Design review of the part shown in the three views and the two pictorial views. Dimensions are in mm from the part's minimum x, y and z. A direction names the side the tool comes from. Round coordinates to 2 decimals unless told otherwise and drop trailing zeros. Order: outer loops, then holes, each group sorted by start corner. A loop starts at its lowest first (then second) coordinate and runs counter-clockwise, first axis right, second up. Notation, with made-up numbers: (0.25, 79.5) - (40.25, 79.5) arc R27 cw to (40.25, 114.5) - close; hole circle Ø3 at (61.25, 9). An arc over 180 degrees is marked (long way). One line per question, with ' | ' between items. Start each with the question number.
Item 1: Add section A-A on z = 20.75. State the section outline as (x, y) points.
Item 2: Add section B-B on y = 96.5. State the section outline as (x, z) points, and give its area (3 significant figures).
Item 3: Add section C-C on x = 111. State the section outline as (y, z) points.
Item 4: Tool access review of the marked faces 1 and 2: name each direction out of +Z, -Z, +X, -X, +Y, -Y from which nothing blocks a thin tool from reaching the whole face with its end or side.
Item 5: Insertion check: pin 1 Ø4 at (x, y) = (143.5, 77.5) entering from +Z; pin 2 Ø8 at (x, z) = (82.5, 9) entering from +Y; pin 3 Ø2 at (x, z) = (116, 1.5) entering from +Y. Each pin has a flat end and moves straight along its axis. Give the tip position at first contact, or say it passes through.
Item 6: For L1, parallel to X at y = 14.5, z = 2.25; L2, parallel to X at y = 124, z = 12.5; L3, parallel to Z at x = 55, y = 111.5, list the stretches that pass through material, from the lowest coordinate up. Write a range as [from, to].
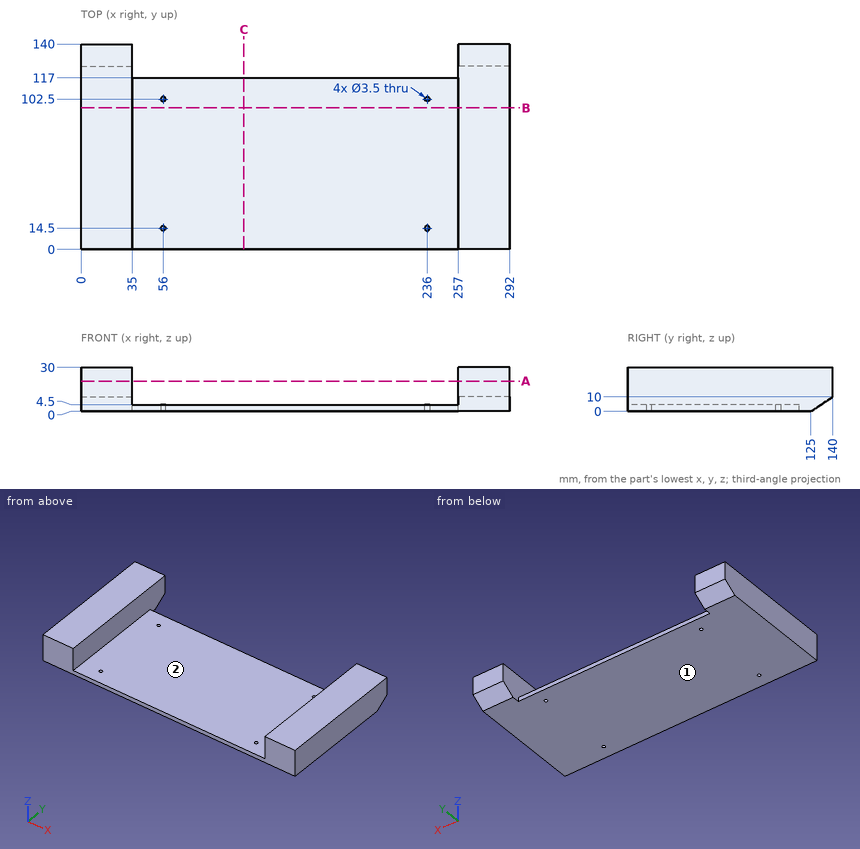
Determined:
1) outline: (0, 0) - (35, 0) - (35, 140) - (0, 140) - close; (257, 0) - (292, 0) - (292, 140) - (257, 140) - close
2) outline: (0, 0) - (292, 0) - (292, 30) - (257, 30) - (257, 4.5) - (35, 4.5) - (35, 30) - (0, 30) - close | area: 3,100 mm2
3) outline: (0, 0) - (117, 0) - (117, 4.5) - (0, 4.5) - close
4) face 1: -Z, +X, -X, +Y, -Y | face 2: +Z, +Y, -Y
5) pin 1: z = 4.5 | pin 2: through | pin 3: y = 117
6) L1: [0, 54.25], [57.75, 234.25], [237.75, 292] | L2: [0, 35], [257, 292] | L3: [0, 4.5]
